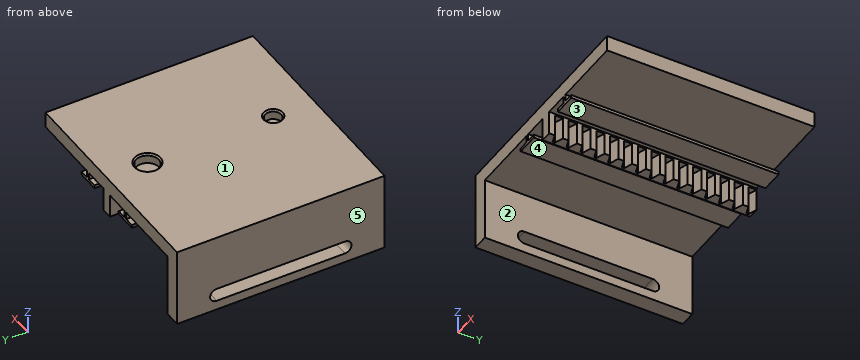
```python
from build123d import *

# Parameters (mm, degrees)
SKETCH_W            = 65.5
SKETCH_H            = 65.5
PAD_DEPTH           = 5
PAD001_DEPTH        = 65.5
SKETCH002_W         = 3.5
SKETCH002_H         = 8
PAD002_DEPTH        = 65.5
POCKET_DEPTH        = 7
LINEARPATTERN_COUNT = 16
LINEARPATTERN_PITCH = 4.366667
SKETCH005_W         = 65.5
SKETCH005_H         = 25
PAD003_DEPTH        = 5
POCKET001_DEPTH     = 5
SKETCH007_R         = 3.6
SKETCH007_R_2       = 2.55
POCKET002_DEPTH     = 3.1
CHAMFER_SIZE        = 0.5


with BuildPart() as part:
    # Sketch → Pad (new body)
    with BuildSketch(Plane.XY):
        Rectangle(SKETCH_W, SKETCH_H)
    extrude(amount=PAD_DEPTH)

    # Sketch001 (on Face3 of Pad) → Pad001 (join)
    with BuildSketch(Plane.XZ.offset(32.75)):
        Polygon((-10.5, 0.5), (-10.5, -2.25), (-13.5, -2.25), (-13.5, -3.25), (-6.5, -3.25), (-6.5, -2.25), (-9.5, -2.25), (-9.5, 0.5), align=None)
        Polygon((9.5, 0.5), (10.5, 0.5), (10.5, -2.25), (13.5, -2.25), (13.5, -3.25), (6.5, -3.25), (6.5, -2.25), (9.5, -2.25), align=None)
    extrude(amount=-PAD001_DEPTH)

    # Sketch002 (on Face1 of Pad001) → Pad002 (join)
    with BuildSketch(Plane(origin=(0, 32.75, 0), x_dir=(-1, 0, 0), z_dir=(0, 1, 0))):
        with Locations((0, -3.5)):
            Rectangle(SKETCH002_W, SKETCH002_H)
    extrude(amount=-PAD002_DEPTH)

    # Sketch003 (on Face32 of Pad002) → Pocket (cut)
    with BuildSketch(Plane(origin=(0, 0, -7.5), x_dir=(1, 0, 0), z_dir=(0, 0, -1))):
        Polygon((1.75, -32.75), (-0.98, -31.795), (-0.98, -31.095), (1.75, -30.14), align=None)
    pocket = extrude(amount=-POCKET_DEPTH, mode=Mode.SUBTRACT)

    # LinearPattern: Pocket ×16
    with Locations(*[(0, -i * LINEARPATTERN_PITCH, 0) for i in range(1, LINEARPATTERN_COUNT)]):
        add(pocket, mode=Mode.SUBTRACT)

    # Sketch005 (on Face11 of LinearPattern) → Pad003 (join)
    with BuildSketch(Plane(origin=(-32.75, 0, 0), x_dir=(0, -1, 0), z_dir=(-1, 0, 0))):
        with Locations((0, -7.5)):
            Rectangle(SKETCH005_W, SKETCH005_H)
    extrude(amount=PAD003_DEPTH)

    # Sketch006 (on Face25 of Pad003) → Pocket001 (cut)
    with BuildSketch(Plane(origin=(-37.75, 0, 0), x_dir=(0, -1, 0), z_dir=(-1, 0, 0))):
        with BuildLine():
            ThreePointArc((-20.25, -12.85), (-22.325, -14.925), (-20.25, -17))
            Line((-20.25, -17), (20.25, -17))
            ThreePointArc((20.25, -17), (22.325, -14.925), (20.25, -12.85))
            Line((20.25, -12.85), (-20.25, -12.85))
        make_face()
    extrude(amount=-POCKET001_DEPTH, mode=Mode.SUBTRACT)

    # Sketch007 (on Face10 of Pocket001) → Pocket002 (cut)
    with BuildSketch(Plane.XY.offset(5)):
        with Locations((0, 19.85)):
            Circle(SKETCH007_R)
        with Locations((0, -19.85)):
            Circle(SKETCH007_R_2)
    extrude(amount=-POCKET002_DEPTH, mode=Mode.SUBTRACT)

    # Chamfer
    chamfer_edges = [part.edges().sort_by_distance(p)[0] for p in [
        (-2.55, -19.85, 5),
        (-3.6, 19.85, 5),
    ]]
    chamfer(chamfer_edges, length=CHAMFER_SIZE)


solid = part.part
```
For this review, take the finished solid that the model builds, in its own axes (mm). Face numbers are marked on the shaded views. A direction names the side the tool comes from. Coordinates: 2 decimals unless noted, no trailing zeros. Write each loop counter-clockwise with the first axis right and the second up, starting at its lowest first coordinate (ties: lowest second). Pieces come first, ordered by that corner, then holes. Notation, with made-up numbers: (-35, 72.5) - (9, 72.5) arc R14 ccw to (9, 85.5) - close; hole circle Ø7 at (85.25, 54). An arc over 180 degrees is marked (long way). Answer in a Markdown table with one row per item. Add a question column.
Q1. Tool access review of the marked faces 1 and 2: name each direction out of +Z, -Z, +X, -X, +Y, -Y from which nothing blocks a thin tool from reaching the whole face with its end or side.
Q2. For P1, Ø0.8, axis at y = 22.5, z = -3, coming from the +X side; P2, Ø7.5, axis at x = -10, y = 9.5, coming from the -Z side; P3, Ø10, axis at x = 1.5, y = 13, coming from the -Z side, all flat-tipped, find the tip position at first contact; note any pin that passes through.
Q3. We need section B-B, the plane x = 28.5. State the section outline as (y, z) points.
Q4. For probe 1 along Y at (x, z) = (0, 3.4); probe 2 along X at (y, z) = (23, -0.25); probe 3 along X at (y, z) = (21, -5), list the stretches that pass through material, from the lowest coordinate up.
Q5. We need section A-A, the plane z = -10. State the section outline as (x, y) points.
Q6. Draft analysis for pull direction X (two halves, no side actions). For the marked faces 3, 4 and 5, state which applies: +X half, -X half, draft (parallel to the pull), parting line (faces both ways), or undercut.
Answer list:
| question | item | result |
|---|---|---|
| 1 | face 1 | +Z, +X, -X, +Y, -Y |
| 1 | face 2 | -Z, +Y, -Y |
| 2 | P1 | stops at x = 13.5 |
| 2 | P2 | stops at z = -3.25 |
| 2 | P3 | stops at z = -7.5 |
| 3 | outline | (-32.75, 0) - (32.75, 0) - (32.75, 5) - (-32.75, 5) - close |
| 4 | probe 1 | y = -32.75 to -22.4, -17.3 to 16.25, 23.45 to 32.75 |
| 4 | probe 2 | x = -37.75 to -32.75, -10.5 to -9.5, -1.75 to 1.75, 9.5 to 10.5 |
| 4 | probe 3 | x = -37.75 to -32.75, -1.75 to 1.75 |
| 5 | outline | (-37.75, -32.75) - (-32.75, -32.75) - (-32.75, 32.75) - (-37.75, 32.75) - close |
| 6 | face 3 | draft |
| 6 | face 4 | undercut |
| 6 | face 5 | -X half |
